Input: part model. Units: mm. Frame: model coordinates. Face numbers are marked on the shaded views. A direction names the side the tool comes from. Give positions to 0.01 mm unless a question says otherwise; leave off trailing zeros. Order: outer loops, then holes, each group sorted by start corner. A loop starts at its lowest first (then second) coordinate and runs counter-clockwise, first axis right, second up. Notation, with made-up numbers: (-32, 65) - (16, 65) arc R19 ccw to (16, 77) - close; hole circle Ø10 at (14.5, 13.25). An arc over 180 degrees is marked (long way). Answer in a Markdown table with one row per item. Add a question column.
1. Section query B-B on z = 2.75. Return loops of the section in (x, y).
2. Section query A-A on y = 0. Return loops of the section in (x, z).
3. Contact query for flat-ended pins moving along their axis: pin 1 (2.5 mm diameter, centred on x = 3, z = 1, fed in from +Y); pin 2 (1.5 mm diameter, centred on x = 5.5, z = -1.5, fed in from -Y); pin 3 (3 mm diameter, centred on x = 8, z = 0.5, fed in from -Y); pin 4 (4.5 mm diameter, centred on x = 7.15, y = 0, fed in from +Z). Output: stop coordinate, or through.
4. Section query D-D on y = 3.5. Return loops of the section in (x, z), and give its area (3 significant figures).
5. Access query for the marked faces 1, 2, 3, 4 and 5. Directions: +Z, -Z, +X, -X, +Y, -Y. A direction counts if a zero-diameter tool reaches every point of the face in a straight line with its end or side. Return the directions, or none.
6. Section query C-C on x = 0. Return loops of the section in (y, z), and give its area (3 significant figures).
7. Ray query, line 1 (Y direction, x = -7.15, z = 0.55); line 2 (Z direction, x = -2.75, y = 2.75); line 3 (X direction, y = 2, z = -1.5). Return the intervals inside material, ascending. Write a range as [from, to].
8. Mould query, pull axis Y, two halves, no side actions, for the marked faces 6, 7, 8 and 9. Classes: released by +Y, released by -Y, zero draft, split by the parting line, or undercut.
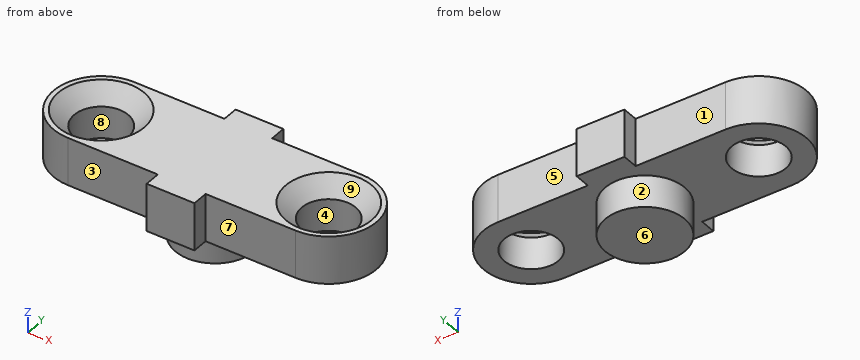
```python
from build123d import *

# Parameters (mm, degrees)
SKETCH1_R           = 1.7
BOSS_EXTRUDE1_DEPTH = 3
CHAMFER1_SIZE       = 1
SKETCH2_R           = 2.5
BOSS_EXTRUDE2_DEPTH = 2


with BuildPart() as part:
    # Sketch1 → Boss-Extrude1 (new body)
    with BuildSketch(Plane.XY):
        with BuildLine():
            Line((-7.15, 3), (-1.5, 3))
            Line((-1.5, 3), (-1.5, 4))
            Line((-1.5, 4), (1.5, 4))
            Line((1.5, 4), (1.5, 3))
            Line((1.5, 3), (7.15, 3))
            ThreePointArc((7.15, 3), (10.15, 0), (7.15, -3))
            Line((7.15, -3), (1.5, -3))
            Line((1.5, -3), (1.5, -4))
            Line((1.5, -4), (-1.5, -4))
            Line((-1.5, -4), (-1.5, -3))
            Line((-1.5, -3), (-7.15, -3))
            ThreePointArc((-7.15, -3), (-10.15, 0), (-7.15, 3))
        make_face()
        with Locations((-7.15, 0)):
            Circle(SKETCH1_R, mode=Mode.SUBTRACT)
        with Locations((7.15, 0)):
            Circle(SKETCH1_R, mode=Mode.SUBTRACT)
    extrude(amount=BOSS_EXTRUDE1_DEPTH)

    # Chamfer1
    chamfer1_edges = [part.edges().sort_by_distance(p)[0] for p in [
        (5.45, 0, 3),
        (-8.85, 0, 3),
    ]]
    chamfer(chamfer1_edges, length=CHAMFER1_SIZE)

    # Sketch2 → Boss-Extrude2 (add)
    with BuildSketch(Plane(origin=(0, 0, 0), x_dir=(-1, 0, 0), z_dir=(0, 0, -1))):
        with Locations(Location((0, 0, 0), (0, 0, 180))):
            Circle(SKETCH2_R)
    extrude(amount=BOSS_EXTRUDE2_DEPTH)


solid = part.part
```
Answer:
| question | item | result |
|---|---|---|
| 1 | outline | (-7.15, -3) - (-1.5, -3) - (-1.5, -4) - (1.5, -4) - (1.5, -3) - (7.15, -3) arc R3 ccw to (7.15, 3) - (1.5, 3) - (1.5, 4) - (-1.5, 4) - (-1.5, 3) - (-7.15, 3) arc R3 ccw to start; hole circle Ø4.9 at (-7.15, 0); hole circle Ø4.9 at (7.15, 0) |
| 2 | outline | (-10.15, 0) - (-8.85, 0) - (-8.85, 2) - (-9.85, 3) - (-10.15, 3) - close; (-5.45, 0) - (-2.5, 0) - (-2.5, -2) - (2.5, -2) - (2.5, 0) - (5.45, 0) - (5.45, 2) - (4.45, 3) - (-4.45, 3) - (-5.45, 2) - close; (8.85, 0) - (10.15, 0) - (10.15, 3) - (9.85, 3) - (8.85, 2) - close |
| 3 | pin 1 | stops at y = 3 |
| 3 | pin 2 | passes through |
| 3 | pin 3 | stops at y = -3 |
| 3 | pin 4 | stops at z = 2.55 |
| 4 | outline | (-1.5, 0) - (1.5, 0) - (1.5, 3) - (-1.5, 3) - close |
| 4 | area | 9.00 mm² |
| 5 | face 1 | +Z, -Z, -X, +Y |
| 5 | face 2 | -Z |
| 5 | face 3 | +Z, -Z, -X, -Y |
| 5 | face 4 | +Z, -Z |
| 5 | face 5 | +Z, -Z, +X, +Y |
| 6 | outline | (-4, 0) - (-2.5, 0) - (-2.5, -2) - (2.5, -2) - (2.5, 0) - (4, 0) - (4, 3) - (-4, 3) - close |
| 6 | area | 34.0 mm² |
| 7 | line 1 | y = [-3, -1.7], [1.7, 3] |
| 7 | line 2 | z = [0, 3] |
| 7 | line 3 | x = [-1.5, 1.5] |
| 8 | face 6 | zero draft |
| 8 | face 7 | released by -Y |
| 8 | face 8 | undercut |
| 8 | face 9 | undercut |
